Could you check a few things on this drawing? It's one solid part, dimensions in mm from its lowest x, y, z. Give positions to 0.01 mm unless a question says otherwise; leave off trailing zeros. Loops run counter-clockwise (first coordinate to the right, second up) from the corner with the lowest first, then second, coordinate; pieces in that order, holes last. Notation, with made-up numbers: (39, 55.5) - (77, 55.5) arc R23 ccw to (77, 87.5) - close; hole circle Ø5 at (68.5, 66.5). An arc over 180 degrees is marked (long way). Answer as a JSON object with one key per item and string values.
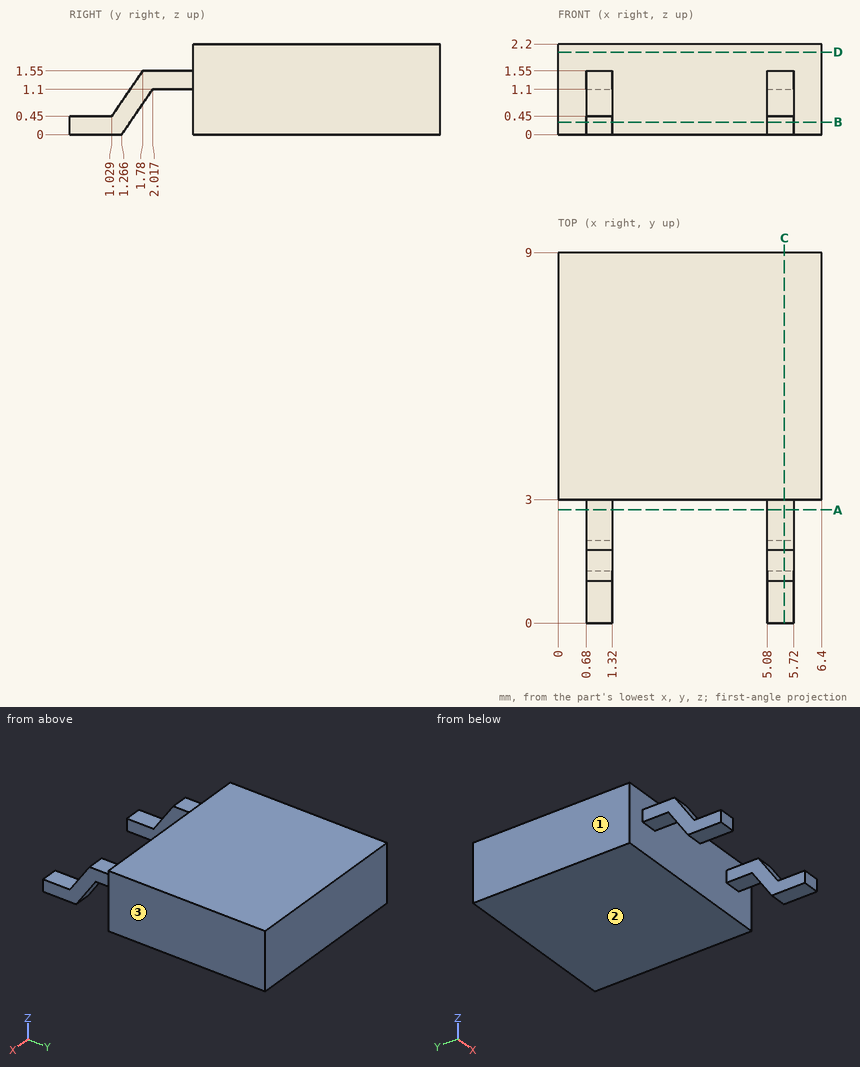
1) Imagine slicing it at D-D on z = 2. Write out the boundary of the cut face in (x, y), and give its area (3 significant figures).
Check sheet entries:
{"outline": "(0, 3) - (6.4, 3) - (6.4, 9) - (0, 9) - close", "area": "38.4 mm2"}
2) Imagine slicing it at C-C on x = 5.5. Write out the boundary of the cut face in (y, z).
Check sheet entries:
{"outline": "(0, 0) - (1.27, 0) - (2.02, 1.1) - (3, 1.1) - (3, 0) - (9, 0) - (9, 2.2) - (3, 2.2) - (3, 1.55) - (1.78, 1.55) - (1.03, 0.45) - (0, 0.45) - close"}
3) Imagine slicing it at B-B on z = 0.3. Write out the boundary of the cut face in (x, y).
Check sheet entries:
{"outline": "(0, 3) - (6.4, 3) - (6.4, 9) - (0, 9) - close; (0.68, 0) - (1.32, 0) - (1.32, 1.47) - (0.68, 1.47) - close; (5.08, 0) - (5.72, 0) - (5.72, 1.47) - (5.08, 1.47) - close"}
4) I need wall thicknesses on L1, parallel to Y at x = 5, z = 0.7; L2, parallel to Z at x = 1, y = 2.5. Which ranges of each line are inside material? Lowest first, please.
Check sheet entries:
{"L1": "3 to 9", "L2": "1.1 to 1.55"}
5) Imagine slicing it at A-A on y = 2.75. Write out the boundary of the cut face in (x, z).
Check sheet entries:
{"outline": "(0.68, 1.1) - (1.32, 1.1) - (1.32, 1.55) - (0.68, 1.55) - close; (5.08, 1.1) - (5.72, 1.1) - (5.72, 1.55) - (5.08, 1.55) - close"}
6) If we mould it in two halves opening along X, with no side actions, what happens to the marked faces 1, 2 and 3? For each: released by +X, released by -X, zero draft, split by the parting line, or undercut.
Check sheet entries:
{"face 1": "released by -X", "face 2": "zero draft", "face 3": "released by +X"}
7) I'm going to push flat-ended pins straight in: P1, Ø0.7, axis at x = 1, y = 2, coming from the +Z side; P2, Ø0.5, axis at y = 1.5, z = 1, coming from the +X side; P3, Ø0.5, axis at x = 1, y = 0.5, coming from the +Z side. Where does each tip first touch, or does it pass through?
Check sheet entries:
{"P1": "z = 1.55", "P2": "x = 5.72", "P3": "z = 0.45"}
